Autodesk Inventor part; units mm, degrees
ref_plane "YZ Plane" through (0, 0, 0) normal (1, 0, 0) x (0, 1, 0)
ref_plane "XZ Plane" through (0, 0, 0) normal (0, 1, 0) x (-1, 0, 0)
ref_plane "XY Plane" through (0, 0, 0) normal (0, 0, 1) x (1, 0, 0)
sketch "Sketch1" plane through (0, 0, 0) normal (0, 1, 0) x (-1, 0, 0)
  line L0 (0, 0) -> (0, -16)
  line L1 (0, -16) -> (2, -16)
  line L2 (0, 0) -> (2, 0)
  line L3 (2, 0) -> (2, -6)
  line L4 (2, -16) -> (2, -13)
  line L5 (2, -13) -> (5, -13)
  line L6 (5, -13) -> (5, -4)
  line L7 (5, -4) -> (2, -6)
  dimension "d0" = 16
  dimension "d1" = 2
  dimension "d2" = 6
  dimension "d3" = 3
  dimension "d4" = 3
  dimension "d5" = 9
extrude "Extrusion1" add sketch "Sketch1" along normal blind 32
sketch "Sketch2" plane through (-5, 0, -13) normal (-1, 0, 0) x (0, 0, 1)
  line L0 (0, 0) -> (9, 0)
  line L1 (9, 0) -> (9, 32)
  line L2 (0, 32) -> (9, 32)
  line L3 (0, 0) -> (0, 32)
  line L4 (0, 0) -> (9, 0)
  line L5 (5.5, 0) -> (5.5, 25)
  line L6 (5.5, 25) -> (0, 25)
  point P0 (13, 0)
  dimension "d8" = 25
  dimension "d9" = 5.5
extrude "Extrusion2" cut sketch "Sketch2" against normal blind 3 contours L3 L6 L5 L0
sketch "Sketch3" plane through (-2, 0, -16) normal (-1, 0, 0) x (0, 0, 1)
  line L0 (0, 0) -> (8.5, 0)
  line L1 (8.5, 25) -> (8.5, 0)
  line L2 (3, 25) -> (8.5, 25)
  line L3 (3, 25) -> (3, 32)
  line L4 (0, 32) -> (3, 32)
  line L5 (0, 0) -> (0, 32)
  line L6 (0, 0) -> (8.5, 0)
  line L7 (0, 0) -> (0, 12)
  line L8 (0, 0) -> (0, 32)
  line L9 (0, 12) -> (3, 12)
  line L10 (3, 12) -> (3, 15)
  line L11 (3, 15) -> (8.5, 15)
  line L12 (8.5, 25) -> (8.5, 0)
  line L13 (3, 25) -> (3, 32)
  line L14 (3, 25) -> (0, 25)
  point P0 (16, 0)
  dimension "d12" = 12
  dimension "d13" = 3
  dimension "d14" = 3
extrude "Extrusion3" cut sketch "Sketch3" against normal blind 4 contours L5 L14 L2 L1 L11 L10 L9
properties part number "Inner Rails 2"
Check sheet for the modelled part. Datum: model origin and axes. Units: mm. A direction names the side the tool comes from. Coordinates: 2 decimals unless noted, no trailing zeros. Write each loop counter-clockwise with the first axis right and the second up, starting at its lowest first coordinate (ties: lowest second). Pieces come first, ordered by that corner, then holes.
Item 1: Access from +Z, -Z, +X, -X, +Y, -Y to the whole of each face (thin tool, end or side, straight path). Record for faces 1 (the face through (-3, 25, -11)), 2 (the face through (-2, 29, -15)), 3 (the face through (-2, 16, -3)).
Numbers:
face 1: -Z, +X, -X
face 2: -Z, -X, +Y, -Y
face 3: +Z, +Y, -Y
Item 2: Cross-section at D-D on z = -9.5. Record the boundary of the cut face in (x, y), then the cut area to 3 significant figures.
Numbers:
outline: (-5, 25) - (0, 25) - (0, 32) - (-5, 32) - close; (-2, 0) - (0, 0) - (0, 15) - (-2, 15) - close
area: 65.0 mm2
Item 3: Cross-section at C-C on x = -1.2. Record the boundary of the cut face in (y, z).
Numbers:
outline: (0, -16) - (12, -16) - (12, -13) - (15, -13) - (15, -7.5) - (25, -7.5) - (25, -16) - (32, -16) - (32, 0) - (0, 0) - close
Item 4: Cross-section at A-A on z = -14.25. Record the boundary of the cut face in (x, y), then the cut area to 3 significant figures.
Numbers:
outline: (-2, 0) - (0, 0) - (0, 12) - (-2, 12) - close; (-2, 25) - (0, 25) - (0, 32) - (-2, 32) - close
area: 38.0 mm2
Item 5: Cross-section at B-B on y = 27. Record the boundary of the cut face in (x, z), then the cut area to 3 significant figures.
Numbers:
outline: (-5, -13) - (-2, -13) - (-2, -16) - (0, -16) - (0, 0) - (-2, 0) - (-2, -6) - (-5, -4) - close
area: 56.0 mm2
Item 6: Scan lines: probe 1 along X at (y, z) = (31.5, -1.75); probe 2 along Y at (x, z) = (-0.2, -13.25); probe 3 along Y at (x, z) = (-4.5, -9). Record each from-to range of solid material in increasing order.
Numbers:
probe 1: x = -2 to 0
probe 2: y = 0 to 12, 25 to 32
probe 3: y = 25 to 32
Item 7: Depth check by flat-ended pin: pin 1 Ø1.5 at (x, z) = (-3.5, -10.5) entering from -Y. Enter the tip coordinate at first touch or a pass-through.
Numbers:
pin 1: stops at y = 25
Item 8: Mould release check, pull along X, two halves, no side actions. Record for faces 4 (the face through (-1, 0, -8)), 5 (the face through (-2, 8, -12)), 6 (the face through (-3.5, 15.8, -5)): released by +X, released by -X, zero draft, split by the parting line, or undercut.
Numbers:
face 4: zero draft
face 5: released by -X
face 6: undercut
